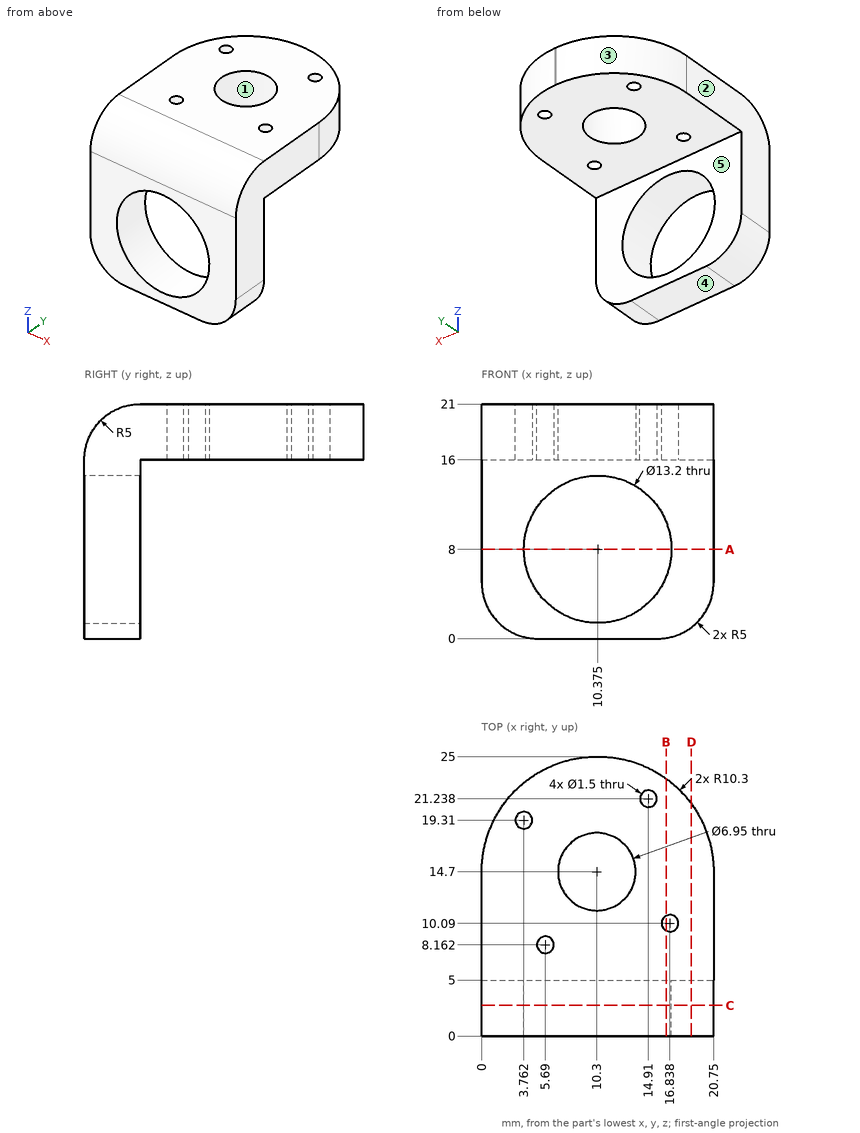
Answer from the drawing. Dimensions are ordinates in mm from the lowest x, y and z of the part. A direction names the side the tool comes from. Coordinates: 2 decimals unless noted, no trailing zeros. Loops run counter-clockwise (first coordinate to the right, second up) from the corner with the lowest first, then second, coordinate; pieces in that order, holes last. Notation, with made-up numbers: (62, 57) - (69, 57) arc R30 ccw to (69, 89) - close; hole circle Ø5 at (6, -18). An arc over 180 degrees is marked (long way). Use a Markdown table: item, result.
Item 1: The mould has two halves that part along Y. Classify the marked faces 1, 2 and 3: +Y half, -Y half, draft (parallel to the pull), parting line (faces both ways), or undercut.
Evaluation:
| item | result |
|---|---|
| face 1 | undercut |
| face 2 | draft |
| face 3 | +Y half |
Item 2: Find section D-D, the plane x = 18.75. Determine the outline of the cut face in (y, z), and give its area (3 significant figures).
Evaluation:
| item | result |
|---|---|
| outline | (0, 1) - (5, 1) - (5, 16) - (20.8, 16) - (20.8, 21) - (5, 21) arc R5 ccw to (0, 16) - close |
| area | 174 mm2 |
Item 3: Find section B-B, the plane x = 16.5. Determine the outline of the cut face in (y, z).
Evaluation:
| item | result |
|---|---|
| outline | (0, 0.06) - (5, 0.06) - (5, 5.54) - (0, 5.54) - close; (0, 10.46) - (5, 10.46) - (5, 16) - (9.42, 16) - (9.42, 21) - (5, 21) arc R5 ccw to (0, 16) - close; (10.76, 16) - (23.04, 16) - (23.04, 21) - (10.76, 21) - close |
Item 4: Consider probe 1 along X at (y, z) = (2, 8) (3 decimals); probe 2 along Z at (x, y) = (15.5, 23.5); probe 3 along Y at (x, z) = (15.75, 1). Determine where each line is inside the solid, lowest interval first. Write a range as from..to.
Evaluation:
| item | result |
|---|---|
| probe 1 | x = 0..3.775, 16.975..20.75 |
| probe 2 | z = 16..21 |
| probe 3 | y = 0..5 |
Item 5: Find section A-A, the plane z = 8. Determine the outline of the cut face in (x, y) (3 decimals).
Evaluation:
| item | result |
|---|---|
| outline | (0, 0) - (3.775, 0) - (3.775, 5) - (0, 5) - close; (16.975, 0) - (20.75, 0) - (20.75, 5) - (16.975, 5) - close |
Item 6: For the marked faces 4 and 5, determine the directions among +Z, -Z, +X, -X, +Y, -Y from which every point of the face is accessible in a straight line to the end or side of a thin tool.
Evaluation:
| item | result |
|---|---|
| face 4 | -Z, +X, -X, +Y, -Y |
| face 5 | -Z, +X, -X, +Y |
Item 7: Given pin 1 Ø1.7 at (x, y) = (5.69, 8.16) entering from +Z; pin 2 Ø10 at (x, y) = (6.5, 16.5) entering from -Z; pin 3 Ø3 at (x, y) = (2, 3.5) entering from -Z; pin 4 Ø6 at (x, z) = (15.5, 12.5) entering from +Y, each flat-ended and moving along its own axis, determine where each tip first touches the part or whether it passes through.
Evaluation:
| item | result |
|---|---|
| pin 1 | stops at z = 21 |
| pin 2 | stops at z = 16 |
| pin 3 | stops at z = 0.23 |
| pin 4 | stops at y = 5 |
Item 8: Find section C-C, the plane y = 2.75. Determine the outline of the cut face in (x, z) (3 decimals), and give its area (3 significant figures).
Evaluation:
| item | result |
|---|---|
| outline | (0, 5) arc R5 ccw to (5, 0) - (15.75, 0) arc R5 ccw to (20.75, 5) - (20.75, 20.465) - (0, 20.465) - close; hole circle Ø13.2 at (10.375, 8) |
| area | 277 mm2 |
